Read the model definition and answer for the solid it produces. Units are mm, in the model's axes. A direction names the side the tool comes from. Round coordinates to 2 decimals unless told otherwise and drop trailing zeros. Write each loop counter-clockwise with the first axis right and the second up, starting at its lowest first coordinate (ties: lowest second). Pieces come first, ordered by that corner, then holes. Notation, with made-up numbers: (-12, 7) - (27, 7) arc R27 ccw to (27, 40) - close; hole circle Ø5 at (8, 18). An arc over 180 degrees is marked (long way). Answer as CSV lines item,"result". Start each with the question number.
1) Find section D-D on x = -34.5. State how many separate pieces and enclosed holes the cut face has, then the cut area to 3 significant figures.
2) Find section C-C on y = 23.5. Determine the outline of the cut face in (x, z), then the cut area to 3 significant figures.
3) Each of these flat-tipped pins is pushed along its axis until it touches: pin 1 (2.5 mm diameter, centred on x = -20.86, z = 20.86, fed in from -Y); pin 2 (5.5 mm diameter, centred on x = -23, y = 27, fed in from +Z); pin 3 (5 mm diameter, centred on y = 6, z = 13, fed in from -X). Where does it stop, or does it pass through?
4) Which of the six approach directions +Z, -Z, +X, -X, +Y, -Y give full straight-line access (tool end or side, diameter ignored) to faces 5 (the cylindrical face through (35.94, 25.9, -4.72)), 6 (the flat face through (0, 5, -29)), 7 (the flat face through (28.3, 18, 5.5)), 8 (the flat face through (-24, 26, -24))?
5) For a pull along Z with two mould halves and no side action, classify faces 1 (the cylindrical face through (28.43, 18.49, -3.73)), 2 (the cylindrical face through (-36, 2, 0)), 3 (the cylindrical face through (31, 2, 0)), 4 (the flat face through (11, 19, 27)) as +Z half, -Z half, draft (parallel to the pull), parting line (faces both ways), or undercut.
6) Find section B-B on x = 0. Determine the outline of the cut face in (y, z), then the cut area to 3 significant figures.
7) Consider line 1 along X through (y, z) = (3.8, 0); line 2 along Y through (x, z) = (-24, 10.5); line 3 along Y through (x, z) = (34, 10.5). Determine where each line is inside the solid, lowest interval first.
from build123d import *

# Parameters (mm, degrees)
SKETCH_1_R          = 38
EXTRUDE_1_DEPTH     = 18
SKETCH_2_R          = 28.672717561
EXTRUDE_2_DEPTH     = 1
SKETCH_3_R          = 36.25
EXTRUDE_3_DEPTH     = 22
FILLET_1_R          = 8
SKETCH_4_R          = 1.5
CUT_EXTRUDE_1_DEPTH = 5
CUT_EXTRUDE_START   = -20
SKETCH_5_W          = 48
SKETCH_5_H          = 10
CUT_EXTRUDE_2_DEPTH = 100


with BuildPart() as part:
    # 草图1 → 凸台-拉伸1 (new body)
    with BuildSketch(Plane(origin=(0, 0, 0), x_dir=(1, 0, 0), z_dir=(0, 1, 0))):
        with Locations(Location((0, 0, 0), (0, 0, 270))):
            Circle(SKETCH_1_R)
    extrude(amount=EXTRUDE_1_DEPTH)

    # 草图2 → 凸台-拉伸2 (add)
    with BuildSketch(Plane(origin=(0, 18, 0), x_dir=(1, 0, 0), z_dir=(0, 1, 0))):
        with Locations(Location((0, 0, 0), (0, 0, 270))):
            Circle(SKETCH_2_R)
    extrude(amount=EXTRUDE_2_DEPTH)

    # 草图3 → 凸台-拉伸3 (add)
    with BuildSketch(Plane(origin=(0, 19, 0), x_dir=(1, 0, 0), z_dir=(0, 1, 0))):
        with Locations(Location((0, 0, 0), (0, 0, 270))):
            Circle(SKETCH_3_R)
    extrude(amount=EXTRUDE_3_DEPTH)

    # 圆角1
    fillet_1_edges = [part.edges().sort_by_distance(p)[0] for p in [
        (0, 41, -36.25),
    ]]
    fillet(fillet_1_edges, radius=FILLET_1_R)

    # 草图4 → 切除-拉伸1 (cut)
    with BuildSketch(Plane.XZ):
        with Locations(Location((-29.5, 0, 0), (0, 0, 270))):
            Circle(SKETCH_4_R)
        with Locations(Location((-20.859650045, 20.859650045, 0), (0, 0, 270))):
            Circle(SKETCH_4_R)
        with Locations(Location((0, 29.5, 0), (0, 0, 270))):
            Circle(SKETCH_4_R)
        with Locations(Location((20.859650045, 20.859650045, 0), (0, 0, 270))):
            Circle(SKETCH_4_R)
        with Locations(Location((-34.5, 0, 0), (0, 0, 270))):
            Circle(SKETCH_4_R)
        with Locations(Location((29.5, 0, 0), (0, 0, 270))):
            Circle(SKETCH_4_R)
        with Locations(Location((20.859650045, -20.859650045, 0), (0, 0, 270))):
            Circle(SKETCH_4_R)
        with Locations(Location((0, -29.5, 0), (0, 0, 270))):
            Circle(SKETCH_4_R)
        with Locations(Location((-20.859650045, -20.859650045, 0), (0, 0, 270))):
            Circle(SKETCH_4_R)
    extrude(amount=-CUT_EXTRUDE_1_DEPTH, mode=Mode.SUBTRACT)

    # 草图5 → 切除-拉伸2 (cut)
    with BuildSketch(Plane(origin=(0, 0, 0), x_dir=(0, 0, -1), z_dir=(1, 0, 0)).offset(CUT_EXTRUDE_START)):
        with Locations((0, 26)):
            Rectangle(SKETCH_5_W, SKETCH_5_H)
    extrude(amount=-CUT_EXTRUDE_2_DEPTH, mode=Mode.SUBTRACT)


solid = part.part
Check values:
1,separate pieces,"3"
1,enclosed holes,"0"
1,area,"736 mm^2"
2,outline,"(-27.17, -24) arc R36.25 ccw (long way) to (-27.17, 24) - (-20, 24) - (-20, -24) - close"
2,area,"3,490 mm^2"
3,pin 1,"stops at y = 5"
3,pin 2,"stops at z = 30.07"
3,pin 3,"stops at x = -36.52"
4,face 5,"+Y"
4,face 6,"-Y"
4,face 7,"none"
4,face 8,"-X"
5,face 1,"parting line"
5,face 2,"undercut"
5,face 3,"undercut"
5,face 4,"draft"
6,outline,"(0, -38) - (18, -38) - (18, -28.67) - (19, -28.67) - (19, -36.25) - (33, -36.25) arc R8 ccw to (41, -28.25) - (41, 28.25) arc R8 ccw to (33, 36.25) - (19, 36.25) - (19, 28.67) - (18, 28.67) - (18, 38) - (0, 38) - (0, 31) - (5, 31) - (5, 28) - (0, 28) - (0, -28) - (5, -28) - (5, -31) - (0, -31) - close"
6,area,"2,960 mm^2"
7,line 1,"x = -38 to -36, -33 to -31, -28 to 28, 31 to 38"
7,line 2,"y = 0 to 21, 31 to 41"
7,line 3,"y = 0 to 18, 19 to 36.19"
